The listing builds one solid part. Answer for the finished solid, in the listing's coordinates (mm). A direction names the side the tool comes from. Coordinates: 2 decimals unless noted, no trailing zeros. Write each loop counter-clockwise with the first axis right and the second up, starting at its lowest first coordinate (ties: lowest second). Pieces come first, ordered by that corner, then holes.
from build123d import *

# Parameters (mm, degrees)
ESQUISSE1_W             = 207
ESQUISSE1_H             = 104
BOSS_EXTRU_1_DEPTH      = 2
ESQUISSE3_R             = 1.5
ENL_V_MAT_EXTRU_1_DEPTH = 3
ESQUISSE4_W             = 9
ESQUISSE4_H             = 33
ESQUISSE4_H_2           = 12
ESQUISSE4_W_2           = 12
ESQUISSE4_H_3           = 9
ESQUISSE4_W_3           = 17.8
BOSS_EXTRU_2_DEPTH      = 10


with BuildPart() as part:
    # Esquisse1 → Boss.-Extru.1 (new body)
    with BuildSketch(Plane(origin=(0, 0, 0), x_dir=(1, 0, 0), z_dir=(0, 1, 0))):
        Rectangle(ESQUISSE1_W, ESQUISSE1_H)
    extrude(amount=BOSS_EXTRU_1_DEPTH)

    # Esquisse3 → Enlèv. mat.-Extru.1 (cut, through all)
    with BuildSketch(Plane(origin=(0, 2, 0), x_dir=(1, 0, 0), z_dir=(0, 1, 0))):
        with Locations((-97.5, 46)):
            Circle(ESQUISSE3_R)
        with Locations((-19.5, 45)):
            Circle(ESQUISSE3_R)
        with Locations((68.3, 44.8)):
            Circle(ESQUISSE3_R)
        with Locations((94.5, 12)):
            Circle(ESQUISSE3_R)
        with Locations((95.5, -44)):
            Circle(ESQUISSE3_R)
        with Locations((-3.5, -41)):
            Circle(ESQUISSE3_R)
        with Locations((-94.5, -44)):
            Circle(ESQUISSE3_R)
    extrude(amount=-ENL_V_MAT_EXTRU_1_DEPTH, mode=Mode.SUBTRACT)

    # Esquisse4 → Boss.-Extru.2 (add)
    with BuildSketch(Plane(origin=(0, 2, 0), x_dir=(1, 0, 0), z_dir=(0, 1, 0))):
        with Locations((-93, 18.5)):
            Rectangle(ESQUISSE4_W, ESQUISSE4_H)
        with Locations((-92, -28)):
            Rectangle(ESQUISSE4_W, ESQUISSE4_H_2)
        with Locations((-72.2, 41.3)):
            Rectangle(ESQUISSE4_W_2, ESQUISSE4_H_3)
        with Locations((-51.6, 41.3)):
            Rectangle(ESQUISSE4_W_3, ESQUISSE4_H_3)
        with Locations((-32.5, 41.3)):
            Rectangle(ESQUISSE4_W_2, ESQUISSE4_H_3)
    extrude(amount=BOSS_EXTRU_2_DEPTH)


solid = part.part
Q1. Given pin 1 (6 mm diameter, centred on y = 9, z = -11, fed in from +X); pin 2 (1.8 mm diameter, centred on x = 68.3, z = -44.8, fed in from +Y); pin 3 (3.5 mm diameter, centred on x = -97.5, z = -46, fed in from -Y); pin 4 (3 mm diameter, centred on x = -35.5, y = 7, fed in from +Z), each flat-ended and moving along its own axis, determine where each tip first touches the part or whether it passes through.
Answers below:
pin 1: stops at x = -88.5
pin 2: passes through
pin 3: stops at y = 0
pin 4: stops at z = -36.8
Q2. The part is cut by section A-A, the plane y = 7.25. Write down the section's boundary in (x, z).
Answers below:
outline: (-97.5, -35) - (-88.5, -35) - (-88.5, -2) - (-97.5, -2) - close; (-96.5, 22) - (-87.5, 22) - (-87.5, 34) - (-96.5, 34) - close; (-78.2, -45.8) - (-66.2, -45.8) - (-66.2, -36.8) - (-78.2, -36.8) - close; (-60.5, -45.8) - (-42.7, -45.8) - (-42.7, -36.8) - (-60.5, -36.8) - close; (-38.5, -45.8) - (-26.5, -45.8) - (-26.5, -36.8) - (-38.5, -36.8) - close
Q3. Which of the six approach directions +Z, -Z, +X, -X, +Y, -Y give full straight-line access (tool end or side, diameter ignored) to faces 1 (the face through (-52, 7, -45.8)), 2 (the face through (-93, 7, -2)), 3 (the face through (-72, 7, -36.8))?
Answers below:
face 1: -Z, +X, -X, +Y
face 2: +X, -X, +Y
face 3: +Z, +X, -X, +Y
Q4. The part is cut by section C-C, the plane x = -32. Write down the section's boundary in (y, z), then the cut area to 3 significant figures.
Answers below:
outline: (0, -52) - (2, -52) - (2, -45.8) - (12, -45.8) - (12, -36.8) - (2, -36.8) - (2, 52) - (0, 52) - close
area: 298 mm2
Q5. The part is cut by section D-D, the plane x = 55. Write down the section's boundary in (y, z), then the cut area to 3 significant figures.
Answers below:
outline: (0, -52) - (2, -52) - (2, 52) - (0, 52) - close
area: 208 mm2
Q6. Determine the mould class of faces 4 (the face through (-66.2, 7, -41)), 5 (the face through (-78.2, 7, -41)), 6 (the face through (-87.5, 7, 28)), 7 (the face through (-72, 12, -41)) for opening direction X: released by +X, released by -X, zero draft, split by the parting line, or undercut.
Answers below:
face 4: undercut
face 5: released by -X
face 6: released by +X
face 7: zero draft
Q7. Find the intervals of material crossed by probe 1 along X at (y, z) = (6, -39); probe 2 along Z at (x, y) = (-19.5, 0.9); probe 3 along X at (y, z) = (1.3, 44), in increasing order.
Answers below:
probe 1: x = -78.2 to -66.2, -60.5 to -42.7, -38.5 to -26.5
probe 2: z = -52 to -46.5, -43.5 to 52
probe 3: x = -103.5 to -96, -93 to 94, 97 to 103.5
Q8. The part is cut by section B-B, the plane z = -8. Write down the section's boundary in (x, y), then the cut area to 3 significant figures.
Answers below:
outline: (-103.5, 0) - (103.5, 0) - (103.5, 2) - (-88.5, 2) - (-88.5, 12) - (-97.5, 12) - (-97.5, 2) - (-103.5, 2) - close
area: 504 mm2
